Read the model definition and answer for the solid it produces. Units are mm, in the model's axes. Give positions to 0.01 mm unless a question says otherwise; leave off trailing zeros. Order: outer loops, then holes, each group sorted by start corner. A loop starts at its lowest first (then second) coordinate and runs counter-clockwise, first axis right, second up. Notation, with made-up numbers: (50.25, -35.5) -> (74.25, -35.5) arc R23 cw to (74.25, -10.5) -> close; hole circle Ø9 at (25, 71). An arc over 180 degrees is marked (long way). Answer as CSV lines item,"result". Start each with the question number.
1) Straight lines are drawn through the part: L1, parallel to Z at x = 74, y = 2.3 (3 decimals); L2, parallel to Y at x = 5.5, z = 35; L3, parallel to Z at x = -69.5, y = 2. For each, find the intervals that lie inside material, in ascending order. Write a range as from..to.
2) Find section B-B (y = 26). Determine the outline of the cut face in (x, z).
3) Find section C-C (x = 0). Determine the outline of the cut face in (y, z) (3 decimals), and give its area (3 significant figures).
4) Find section A-A (x = 74). Determine the outline of the cut face in (y, z) (3 decimals).
5) Flat-ended cylindrical pins translate along their axes: pin 1 Ø2.5 at (y, z) = (1.5, 128) entering from -X; pin 2 Ø0.9 at (y, z) = (1.5, 5) entering from +X; pin 3 Ø3 at (x, z) = (-74, 6.675) entering from -Y; pin 4 Ø3 at (x, y) = (1.5, 25.5) entering from -Z. Find the tip coordinate at first contact, or state that the pin passes through.
6) Find section D-D (z = 54). Determine the outline of the cut face in (x, y).
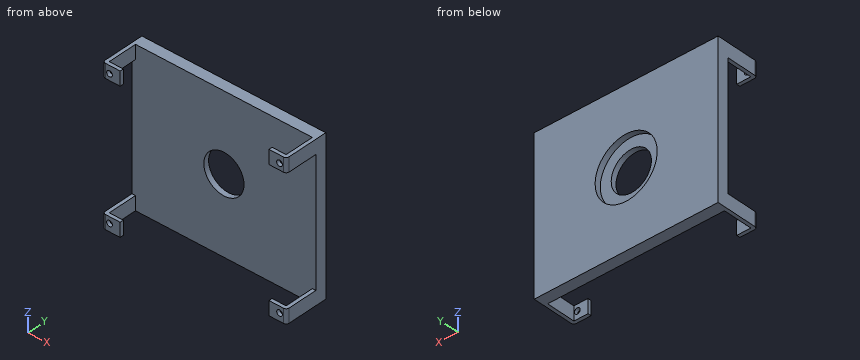
```python
from build123d import *

# Parameters (mm, degrees)
BOSS_EXTRU_1_DEPTH      = 133.35
ESQUISSE3_W             = 108.966
ESQUISSE3_H             = 28.58
ENL_V_MAT_EXTRU_1_DEPTH = 212.421528942
CONG_1_R                = 2.54
SKETCH1_W               = 160.02
SKETCH1_H               = 133.35
BOSS_EXTRUDE1_DEPTH     = 2
SKETCH2_R               = 17.5
CUT_EXTRUDE1_DEPTH      = 161.134514081
SKETCH2_3_R             = 27
SKETCH2_3_R_2           = 17.5
CUT_EXTRUDE2_DEPTH      = 5
SKETCH3_R               = 2.5
CUT_EXTRUDE3_DEPTH      = 5


with BuildPart() as part:
    # Esquisse2 → Boss.-Extru.1 (new body)
    with BuildSketch(Plane.XY):
        Polygon((-64.77, 0), (-80.01, 0), (-80.01, 36.2), (80.01, 36.2), (80.01, 0), (64.77, 0), (64.77, 3.048), (76.962, 3.048), (76.962, 28.58), (-76.962, 28.58), (-76.962, 3.048), (-64.77, 3.048), align=None)
    extrude(amount=BOSS_EXTRU_1_DEPTH)

    # Esquisse3 → Enl_v. mat.-Extru.1 (cut, through all)
    with BuildSketch(Plane.ZY.offset(80.01)):
        with Locations((66.675, 14.29)):
            Rectangle(ESQUISSE3_W, ESQUISSE3_H)
    extrude(amount=-ENL_V_MAT_EXTRU_1_DEPTH, mode=Mode.SUBTRACT)

    # Cong_1
    cong_1_edges = [part.edges().sort_by_distance(p)[0] for p in [
        (-80.01, 0, 127.254),
        (80.01, 0, 127.254),
        (-80.01, 0, 6.096),
        (80.01, 0, 6.096),
    ]]
    fillet(cong_1_edges, radius=CONG_1_R)

    # Sketch1 → Boss-Extrude1 (add)
    with BuildSketch(Plane(origin=(0, 36.2, 0), x_dir=(1, 0, 0), z_dir=(0, 1, 0))):
        with Locations((0, -66.675)):
            Rectangle(SKETCH1_W, SKETCH1_H)
    extrude(amount=BOSS_EXTRUDE1_DEPTH)

    # Sketch2 → Cut-Extrude1 (cut, through all)
    with BuildSketch(Plane(origin=(0, 38.2, 0), x_dir=(1, 0, 0), z_dir=(0, 1, 0))):
        with Locations(Location((0, -66.675, 0), (0, 0, 270))):
            Circle(SKETCH2_R)
    extrude(amount=-CUT_EXTRUDE1_DEPTH, mode=Mode.SUBTRACT)

    # Sketch2_3 → Cut-Extrude2 (cut)
    with BuildSketch(Plane(origin=(0, 38.2, 0), x_dir=(1, 0, 0), z_dir=(0, 1, 0))):
        with Locations(Location((0, -66.675, 0), (0, 0, 270))):
            Circle(SKETCH2_3_R)
        with Locations(Location((0, -66.675, 0), (0, 0, 270))):
            Circle(SKETCH2_3_R_2, mode=Mode.SUBTRACT)
    extrude(amount=-CUT_EXTRUDE2_DEPTH, mode=Mode.SUBTRACT)

    # Sketch3 → Cut-Extrude3 (cut)
    with BuildSketch(Plane.XZ):
        with Locations((-74, 126.675)):
            Circle(SKETCH3_R)
        with Locations((74, 126.675)):
            Circle(SKETCH3_R)
        with Locations((74, 6.675)):
            Circle(SKETCH3_R)
        with Locations((-74, 6.675)):
            Circle(SKETCH3_R)
    extrude(amount=-CUT_EXTRUDE3_DEPTH, mode=Mode.SUBTRACT)


solid = part.part
```
Findings below:
1,L1,"0..4.175, 9.175..12.192, 121.158..124.175, 129.175..133.35"
1,L2,"28.58..38.2"
1,L3,"0..12.19, 121.16..133.35"
2,outline,"(-80.01, 0) -> (-76.96, 0) -> (-76.96, 12.19) -> (-80.01, 12.19) -> close; (-80.01, 121.16) -> (-76.96, 121.16) -> (-76.96, 133.35) -> (-80.01, 133.35) -> close; (76.96, 0) -> (80.01, 0) -> (80.01, 12.19) -> (76.96, 12.19) -> close; (76.96, 121.16) -> (80.01, 121.16) -> (80.01, 133.35) -> (76.96, 133.35) -> close"
3,outline,"(28.58, 0) -> (38.2, 0) -> (38.2, 39.675) -> (33.2, 39.675) -> (33.2, 49.175) -> (28.58, 49.175) -> close; (28.58, 84.175) -> (33.2, 84.175) -> (33.2, 93.675) -> (38.2, 93.675) -> (38.2, 133.35) -> (28.58, 133.35) -> close"
3,area,"851 mm²"
4,outline,"(0, 0) -> (3.048, 0) -> (3.048, 4.175) -> (0, 4.175) -> close; (0, 9.175) -> (3.048, 9.175) -> (3.048, 12.192) -> (0, 12.192) -> close; (0, 121.158) -> (3.048, 121.158) -> (3.048, 124.175) -> (0, 124.175) -> close; (0, 129.175) -> (3.048, 129.175) -> (3.048, 133.35) -> (0, 133.35) -> close; (28.58, 0) -> (38.2, 0) -> (38.2, 133.35) -> (28.58, 133.35) -> close"
5,pin 1,"x = -80.01"
5,pin 2,"x = 79.94"
5,pin 3,"y = 28.58"
5,pin 4,"through"
6,outline,"(-80.01, 28.58) -> (-12.07, 28.58) -> (-12.07, 33.2) -> (-23.84, 33.2) -> (-23.84, 38.2) -> (-80.01, 38.2) -> close; (12.07, 28.58) -> (80.01, 28.58) -> (80.01, 38.2) -> (23.84, 38.2) -> (23.84, 33.2) -> (12.07, 33.2) -> close"
